Geometry check sheet. Reference: the model listing, model coordinates, mm. Face numbers are marked on the shaded views. A direction names the side the tool comes from. Round coordinates to 2 decimals unless told otherwise and drop trailing zeros. Write each loop counter-clockwise with the first axis right and the second up, starting at its lowest first coordinate (ties: lowest second). Pieces come first, ordered by that corner, then holes. Notation, with made-up numbers: (1, 28.25) -> (30, 28.25) arc R14 ccw to (30, 42.25) -> close; hole circle Ø11 at (52, -27). An arc over 180 degrees is marked (long way). One line per question, with ' | ' between items.
```python
from build123d import *

# Parameters (mm, degrees)
BOSS_EXTRUDE2_DEPTH = 40
CUT_EXTRUDE1_DEPTH  = 40


with BuildPart() as part:
    # Sketch1 → Boss-Extrude2 (new body)
    with BuildSketch(Plane(origin=(0, 0, 0), x_dir=(1, 0, 0), z_dir=(0, 1, 0))):
        Polygon((32.948717949, 4.188034188), (-17.051282051, 4.188034188), (-17.051282051, -15.811965812), (-2.051282051, -15.811965812), (-2.051282051, -35.811965812), (17.948717949, -35.811965812), (17.948717949, -15.811965812), (32.948717949, -15.811965812), align=None)
    extrude(amount=-BOSS_EXTRUDE2_DEPTH)

    # Sketch3 → Cut-Extrude1 (cut)
    with BuildSketch(Plane(origin=(0, 0, 0), x_dir=(1, 0, 0), z_dir=(0, 1, 0))):
        Polygon((27.948717949, -0.811965812), (-12.051282051, -0.811965812), (-12.051282051, -10.811965812), (2.948717949, -10.811965812), (2.948717949, -30.811965812), (12.948717949, -30.811965812), (12.948717949, -10.811965812), (27.948717949, -10.811965812), align=None)
    extrude(amount=-CUT_EXTRUDE1_DEPTH, mode=Mode.SUBTRACT)


solid = part.part
```
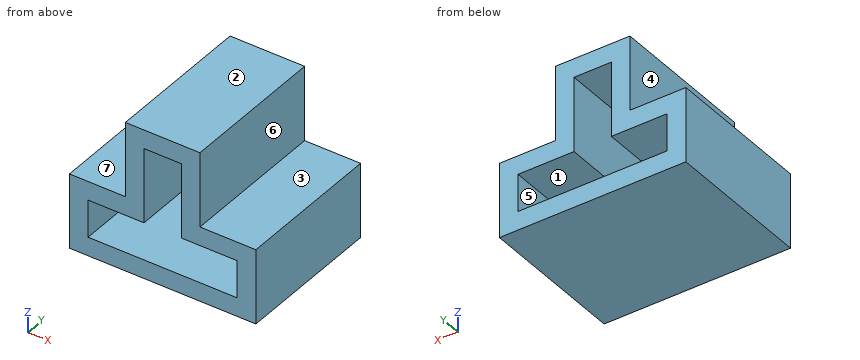
(1) Sectioned sample at B-B on x = 2. Record the cut outline in (y, z).
Resolved:
outline: (-40, -4.19) -> (0, -4.19) -> (0, 0.81) -> (-40, 0.81) -> close; (-40, 10.81) -> (0, 10.81) -> (0, 35.81) -> (-40, 35.81) -> close
(2) Material ranges on line 1 (Z direction, x = -1.5, y = -26.5); line 2 (X direction, y = -2, z = 18); line 3 (Z direction, x = 9, y = -3.5), recorded low to high.
Resolved:
line 1: z = -4.19 to 0.81, 10.81 to 35.81 | line 2: x = -2.05 to 2.95, 12.95 to 17.95 | line 3: z = -4.19 to 0.81, 30.81 to 35.81
(3) Go/stop test with flat-tipped pins: pin 1 (6 mm diameter, centred on y = -16.5, z = 27.5, fed in from -X); pin 2 (4.5 mm diameter, centred on x = -6, y = -21.5, fed in from +Z); pin 3 (3 mm diameter, centred on y = -28.5, z = 21.5, fed in from +X); pin 4 (6 mm diameter, centred on x = -5.5, z = 31, fed in from +Y). Record where each tip stops, or that it passes through.
Resolved:
pin 1: stops at x = -2.05 | pin 2: stops at z = 15.81 | pin 3: stops at x = 17.95 | pin 4: passes through
(4) Access from +Z, -Z, +X, -X, +Y, -Y to the whole of each face (thin tool, end or side, straight path). Record for the marked faces 1, 2, 3 and 4.
Resolved:
face 1: +Y, -Y | face 2: +Z, +X, -X, +Y, -Y | face 3: +Z, +X, +Y, -Y | face 4: +Z, -X, +Y, -Y
(5) Sectioned sample at A-A on z = 21.5. Record the cut outline in (x, y).
Resolved:
outline: (-2.05, -40) -> (2.95, -40) -> (2.95, 0) -> (-2.05, 0) -> close; (12.95, -40) -> (17.95, -40) -> (17.95, 0) -> (12.95, 0) -> close
(6) Draft check along X on the marked faces 5, 6 and 7. Enter one of: +X half, -X half, draft (parallel to the pull), parting line (faces both ways), or undercut.
Resolved:
face 5: undercut | face 6: +X half | face 7: draft
(7) Sectioned sample at C-C on y = -34. Record the cut outline in (x, z).
Resolved:
outline: (-17.05, -4.19) -> (32.95, -4.19) -> (32.95, 15.81) -> (17.95, 15.81) -> (17.95, 35.81) -> (-2.05, 35.81) -> (-2.05, 15.81) -> (-17.05, 15.81) -> close; hole (-12.05, 0.81) -> (27.95, 0.81) -> (27.95, 10.81) -> (12.95, 10.81) -> (12.95, 30.81) -> (2.95, 30.81) -> (2.95, 10.81) -> (-12.05, 10.81) -> close
